```python
from build123d import *

# Parameters (mm, degrees)
SALIENTE_EXTRUIR1_DEPTH = 30
REDONDEO1_R             = 5
CROQUIS2_R              = 2
CORTAR_EXTRUIR1_DEPTH   = 41.197257902


with BuildPart() as part:
    # Croquis1 → Saliente-Extruir1 (new body)
    with BuildSketch(Plane(origin=(0, 0, 0), x_dir=(0, 0, -1), z_dir=(1, 0, 0))):
        with BuildLine():
            Line((-172, 0), (-168, 0))
            ThreePointArc((-168, 0), (-167.590760444, 11.719087589), (-166.365035549, 23.381080961))
            Line((-166.365035549, 23.381080961), (-170.326107824, 23.937773365))
            ThreePointArc((-170.326107824, 23.937773365), (-171.581016645, 11.998113484), (-172, 0))
        make_face()
    extrude(amount=SALIENTE_EXTRUIR1_DEPTH)

    # Redondeo1
    # the kernel refuses this fillet: 5 mm, written as the material it takes off along each edge
    with BuildSketch(Plane(origin=(-11.928000159, 0, 168), x_dir=(0, 0, 1), z_dir=(1, 0, 0))) as redondeo1_piece_1:
        with BuildLine():
            CenterArc((4.930232558, -4.912704692), REDONDEO1_R, 100.722152416, 77.650592735)
            Line((-0.067751042, -4.770719007), (-0.167710714, -4.767879293))
            ThreePointArc((-0.167710714, -4.767879293), (-0.116928532, -2.384180032), (-0.1, 0))
            Line((-0.1, 0), (0, 0.1))
            ThreePointArc((0, 0.1), (2, 0.1), (3.981395349, 0.098254094))
            Line((3.981395349, 0.098254094), (4, 0))
        make_face()
    redondeo1_piece_1_solid = extrude(amount=53.856000318, mode=Mode.PRIVATE)
    with BuildSketch(Plane(origin=(0, 0, 0), x_dir=(0, -0.07283715429145175, 0.9973438469027236), z_dir=(0, -0.9973438469027236, -0.07283715429145175))) as redondeo1_piece_2:
        with BuildLine():
            CenterArc((173, -4.898979486), REDONDEO1_R, 101.536959033, 78.463040967)
            Line((172, 0), (171.98, 0.09797959))
            ThreePointArc((171.98, 0.09797959), (170, 0.1), (168, 0.1))
            Line((168, 0.1), (167.9, 0))
            Line((167.9, 0), (167.9, -4.898979486))
            Line((167.9, -4.898979486), (168, -4.898979486))
        make_face()
    redondeo1_piece_2_solid = revolve(axis=Axis((0, 0, 0), (-1, 0, 0)), revolution_arc=16.353920807, mode=Mode.PRIVATE)
    with BuildSketch(Plane(origin=(-11.928000159, 23.381080961, 166.365035549), x_dir=(0, -0.9921444829388189, 0.12509726205662378), z_dir=(1, 0, 0))) as redondeo1_piece_3:
        with BuildLine():
            CenterArc((4.842200065, -4.999495875), REDONDEO1_R, 90.813627425, 77.650592735)
            Line((-0.056800001, -3.9995967), (-0.154780002, -3.979598716))
            ThreePointArc((-0.154780002, -3.979598716), (-0.128389918, -1.99837835), (-0.099989917, 0.00142))
            Line((-0.099989917, 0.00142), (0.00142, 0.099989917))
            ThreePointArc((0.00142, 0.099989917), (2.385600032, 0.083061386), (4.769780064, 0.099989917))
            Line((4.769780064, 0.099989917), (4.771200064, 0))
        make_face()
    redondeo1_piece_3_solid = extrude(amount=53.856000318, mode=Mode.PRIVATE)
    add([redondeo1_piece_1_solid, redondeo1_piece_2_solid, redondeo1_piece_3_solid], mode=Mode.SUBTRACT)

    # Croquis2 → Cortar-Extruir1 (cut, through all)
    with BuildSketch(Plane.XY.offset(160.05)):
        with Locations(Location((18, 15, 0), (0, 0, 180))):
            Circle(CROQUIS2_R)
        with Locations(Location((12, 15, 0), (0, 0, 180))):
            Circle(CROQUIS2_R)
        with Locations(Location((18, 9, 0), (0, 0, 180))):
            Circle(CROQUIS2_R)
        with Locations(Location((12, 9, 0), (0, 0, 180))):
            Circle(CROQUIS2_R)
    extrude(amount=CORTAR_EXTRUIR1_DEPTH, mode=Mode.SUBTRACT)


solid = part.part
```
Check sheet for the modelled part. Datum: model origin and axes. Units: mm. Give positions to 0.01 mm unless a question says otherwise; leave off trailing zeros. Order: outer loops, then holes, each group sorted by start corner. A loop starts at its lowest first (then second) coordinate and runs counter-clockwise, first axis right, second up. Notation, with made-up numbers: M 25,4.5 L 51,4.5 A9 ccw 51,11.5 Z; hole C -22.5,-27.5 d11. An arc over 180 degrees is marked long. Answer in a Markdown table with one row per item.
1) Cross-section at B-B, the plane x = 9. Enter the section's corners in (y, z).
Filled sheet:
| item | result |
|---|---|
| outline | M 0,172 A5 ccw 4.77,167.93 A168 cw 18.65,166.96 A5 ccw 23.94,170.33 A172 ccw Z |
2) Release check for a two-part mould opening along Y. For faces 1 (the cylindrical face through (17.3, 11.6, 167.6)), 2 (the flat face through (30, 12, 170)), 3 (the cylindrical face through (12, 17, 169)) record: +Y half, -Y half, draft (parallel to the pull), parting line (faces both ways), or undercut.
Filled sheet:
| item | result |
|---|---|
| face 1 | -Y half |
| face 2 | draft |
| face 3 | undercut |
3) Thickness scan on L1, parallel to Y at x = 12.5, z = 169.95; L2, parallel to X at y = 15, z = 168.3; L3, parallel to Y at x = 18, z = 168.85. Record the ranges inside material, lowest first. Write a range as [from, to].
Filled sheet:
| item | result |
|---|---|
| L1 | y = [0.9, 7.06], [10.94, 13.06], [16.94, 23.79] |
| L2 | x = [1.94, 10], [14, 16], [20, 30] |
| L3 | y = [2.02, 7], [11, 13], [17, 23.14] |
4) Gauge pin test, flat ends, axial feed: P1, Ø3, axis at x = 15.5, y = 7, coming from the -Z side; P2, Ø1, axis at x = 6.5, z = 168.5, coming from the +Y side; P3, Ø4.5, axis at x = 12, y = 9, coming from the -Z side; P4, Ø2.5, axis at x = 12, y = 15, coming from the -Z side. Record the tip position at first contact, or that the pin passes through.
Filled sheet:
| item | result |
|---|---|
| P1 | stops at z = 167.78 |
| P2 | stops at y = 23.25 |
| P3 | stops at z = 167.62 |
| P4 | passes through |
5) Cross-section at A-A, the plane x = 19. Enter the section's corners in (y, z), plus the area to 3 significant figures.
Filled sheet:
| item | result |
|---|---|
| outline | M 0,172 A5 ccw 4.77,167.93 A168 cw 7.27,167.84 L 7.27,171.85 A172 ccw Z; M 10.73,167.66 A168 cw 13.27,167.48 L 13.27,171.49 A172 ccw 10.73,171.66 Z; M 16.73,167.16 A168 cw 18.65,166.96 A5 ccw 23.94,170.33 A172 ccw 16.73,171.18 Z |
| area | 57.6 mm2 |
6) Cross-section at C-C, the plane y = 9. Count the separate pieces of the cut face and the enclosed holes in it, plus the area to 3 significant figures.
Filled sheet:
| item | result |
|---|---|
| separate pieces | 3 |
| enclosed holes | 0 |
| area | 83.2 mm2 |
